```python
from build123d import *

# Parameters (mm, degrees)
F0_W     = 31.75
F0_H     = 7.9375
F0_R     = 2.38125
F1_DEPTH = 9.525
F2_DEPTH = 11.1125
F3_T     = -1.5875
F4_R     = 1.5875
F4_R_2   = 0.79375
F5_DEPTH = 7.9375


# Not quite as in the source:
# - a feature names something its author has since deleted; it is built from what else it names


with BuildPart() as f1:
    # F0 (on Top) → F1 (new body)
    with BuildSketch(Plane.XY):
        Rectangle(F0_W, F0_H)
        with Locations((-11.90625, 0)):
            Circle(F0_R, mode=Mode.SUBTRACT)
        with Locations((-3.96875, 0)):
            Circle(F0_R, mode=Mode.SUBTRACT)
        with Locations((3.96875, 0)):
            Circle(F0_R, mode=Mode.SUBTRACT)
        with Locations((11.90625, 0)):
            Circle(F0_R, mode=Mode.SUBTRACT)
    extrude(amount=F1_DEPTH)

    # F0 (on Top) → F2 (join)
    with BuildSketch(Plane.XY):
        with Locations((-11.90625, 0)):
            Circle(F0_R)
        with Locations((-3.96875, 0)):
            Circle(F0_R)
        with Locations((3.96875, 0)):
            Circle(F0_R)
        with Locations((11.90625, 0)):
            Circle(F0_R)
    extrude(amount=F2_DEPTH)

    # F3
    f3_openings = [f1.faces().sort_by_distance(p)[0] for p in [
        (0, 0, 0),
    ]]
    offset(amount=F3_T, openings=f3_openings, kind=Kind.INTERSECTION)

    # F4 (on face) → F5 (join)
    with BuildSketch(Plane(origin=(0, 0, 7.9375), x_dir=(1, 0, 0), z_dir=(0, 0, -1))):
        with Locations((-7.9375, 0)):
            Circle(F4_R)
        with Locations((-7.9375, 0)):
            Circle(F4_R_2, mode=Mode.SUBTRACT)
        Circle(F4_R)
        Circle(F4_R_2, mode=Mode.SUBTRACT)
        with Locations((7.9375, 0)):
            Circle(F4_R)
        with Locations((7.9375, 0)):
            Circle(F4_R_2, mode=Mode.SUBTRACT)
    extrude(amount=F5_DEPTH)


solid = f1.part
```
Could you check a few things on this model? Use its own coordinates, in mm. A direction names the side the tool comes from. Round coordinates to 2 decimals unless told otherwise and drop trailing zeros. Write each loop counter-clockwise with the first axis right and the second up, starting at its lowest first coordinate (ties: lowest second). Pieces come first, ordered by that corner, then holes. Notation, with made-up numbers: M -31,-1.5 L -13,-1.5 A16 ccw -13,20.5 Z; hole C 46,62.25 d9. An arc over 180 degrees is marked long. Write each question's results on one line, items separated by ' | '. Start each with the question number.
1. I need wall thicknesses on L1, parallel to X at y = 0, z = 8.75 (1 decimal); L2, parallel to Y at x = 0, z = 4.5; L3, parallel to Y at x = -14, z = 0.5. Which ranges of each line are inside material? Lowest first, please. Write a range as from..to.
2. Imagine slicing it at D-D on x = 11.5. List the corners of the cut face in (y, z) for me (1 decimal).
3. Imagine slicing it at C-C on y = 3. List the corners of the cut face in (x, z) for me (3 decimals), and give its area (3 significant figures).
4. I'm going to push flat-ended pins straight in: pin 1 Ø1.3 at (x, y) = (-12, 0) entering from -Z (3 decimals); pin 2 Ø1.5 at (x, y) = (-4.5, 0) entering from -Z. Where does each tip first touch, or does it pass through?
5. Imagine slicing it at B-B on x = 0. List the corners of the cut face in (y, z) for me (1 decimal).
6. Thinking about a two-plate mould opening in X: for faces 4 (the face through (-15.875, 0, 5)), 5 (the face through (12, 0, 11.112)), 6 (the face through (9.45, -0.48, 4.02)), which applies, +X half, -X half, draft (parallel to the pull), parting line (faces both ways), or undercut?
7. On a 3-axis mill with a long thin cutter (end or side, diameter ignored), from which of +Z, -Z, +X, -X, +Y, -Y can I reach the whole of each face in a straight line? I mean faces 1 (the face through (8, 0, 7.938)), 2 (the face through (-12, 0, 11.112)), 3 (the face through (0, 0, 9.525)). Say none if no direction works.
8. Imagine slicing it at A-A on z = 5.5. Count the separate pieces of the cut face and the enclosed holes in it, and give its area (3 significant figures).
Result sheet:
1) L1: x = -15.9..-12.7, -11.1..-4.8, -3.2..3.2, 4.8..11.1, 12.7..15.9 | L2: y = -3.97..-2.38, -1.59..-0.79, 0.79..1.59, 2.38..3.97 | L3: y = -3.97..-2.38, 2.38..3.97
2) outline: M -4,0 L -2.4,0 L -2.4,7.9 L -0.7,7.9 L -0.7,9.5 L 0.7,9.5 L 0.7,7.9 L 2.4,7.9 L 2.4,0 L 4,0 L 4,9.5 L 2.3,9.5 L 2.3,11.1 L -2.3,11.1 L -2.3,9.5 L -4,9.5 Z
3) outline: M -15.875,0 L 15.875,0 L 15.875,9.525 L -15.875,9.525 Z | area: 302 mm^2
4) pin 1: stops at z = 9.525 | pin 2: stops at z = 7.94
5) outline: M -4,0 L -2.4,0 L -2.4,7.9 L -1.6,7.9 L -1.6,0 L -0.8,0 L -0.8,7.9 L 0.8,7.9 L 0.8,0 L 1.6,0 L 1.6,7.9 L 2.4,7.9 L 2.4,0 L 4,0 L 4,9.5 L -4,9.5 Z
6) face 4: -X half | face 5: draft | face 6: undercut
7) face 1: -Z | face 2: +Z, +X, -X, +Y, -Y | face 3: +Z
8) separate pieces: 4 | enclosed holes: 4 | area: 134 mm^2
